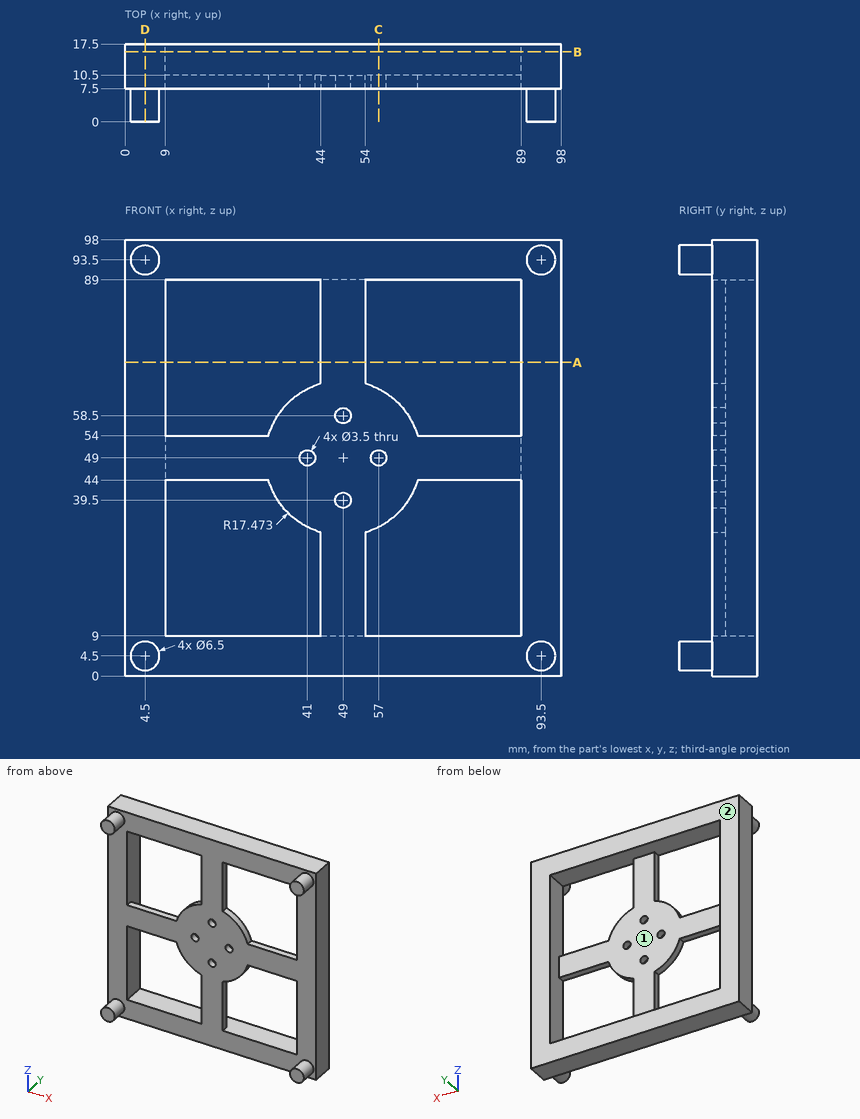
The figure shows three views and two pictorial views of one solid part (mm, origin at its lowest corner). Answer the questions. Give positions to 0.01 mm unless a question says otherwise; leave off trailing zeros. Order: outer loops, then holes, each group sorted by start corner. A loop starts at its lowest first (then second) coordinate and runs counter-clockwise, first axis right, second up. Notation, with made-up numbers: (-10, 35.5) -> (46, 35.5) arc R27 ccw to (46, 70.5) -> close; hole circle Ø2 at (39, 77). An arc over 180 degrees is marked (long way). Answer as a JSON object with one key per item and string values. Group by question number.
Item 1: Consider L1, parallel to X at y = 9.5, z = 49; L2, parallel to X at y = 9.25, z = 72; L3, parallel to X at y = 12.5, z = 47. Determine where each line is inside the solid, lowest interval first. Write a range as from..to.
Item 2: Determine the mould class of the marked faces 1 and 2 for opening direction X: pulls with the +X half, pulls with the -X half, needs draft (parallel to the pull), parting line crosses it, or undercut.
Item 3: The part is cut by section B-B on y = 15.75. Write down the section's boundary in (x, z), and give its area (3 significant figures).
Item 4: Flat-ended cylindrical pins translate along their axes: pin 1 (0.9 mm diameter, centred on x = 77.5, y = 9.5, fed in from -Z); pin 2 (4 mm diameter, centred on x = 49, z = 39.5, fed in from -Y). Find the tip coordinate at first contact, or state that the pin passes through.
Item 5: The part is cut by section C-C on x = 57. Write down the section's boundary in (y, z).
Item 6: The part is cut by section D-D on x = 4.5. Write down the section's boundary in (y, z), and give its area (3 significant figures).
Item 7: The part is cut by section A-A on z = 70.5. Write down the section's boundary in (x, y), and give its area (3 significant figures).
Result set:
{
 "1": {"L1": "0..39.25, 42.75..55.25, 58.75..98", "L2": "0..9, 44..54, 89..98", "L3": "0..9, 89..98"},
 "2": {"face 1": "undercut", "face 2": "needs draft"},
 "3": {"outline": "(0, 0) -> (98, 0) -> (98, 98) -> (0, 98) -> close; hole (9, 9) -> (89, 9) -> (89, 89) -> (9, 89) -> close", "area": "3,200 mm²"},
 "4": {"pin 1": "z = 0", "pin 2": "y = 7.5"},
 "5": {"outline": "(7.5, 0) -> (17.5, 0) -> (17.5, 9) -> (7.5, 9) -> close; (7.5, 33.47) -> (10.5, 33.47) -> (10.5, 47.25) -> (7.5, 47.25) -> close; (7.5, 50.75) -> (10.5, 50.75) -> (10.5, 64.53) -> (7.5, 64.53) -> close; (7.5, 89) -> (17.5, 89) -> (17.5, 98) -> (7.5, 98) -> close"},
 "6": {"outline": "(0, 1.25) -> (7.5, 1.25) -> (7.5, 0) -> (17.5, 0) -> (17.5, 98) -> (7.5, 98) -> (7.5, 96.75) -> (0, 96.75) -> (0, 90.25) -> (7.5, 90.25) -> (7.5, 7.75) -> (0, 7.75) -> close", "area": "1,080 mm²"},
 "7": {"outline": "(0, 7.5) -> (9, 7.5) -> (9, 17.5) -> (0, 17.5) -> close; (44, 7.5) -> (54, 7.5) -> (54, 10.5) -> (44, 10.5) -> close; (89, 7.5) -> (98, 7.5) -> (98, 17.5) -> (89, 17.5) -> close", "area": "210 mm²"}
}
